For this review, use the dimensioned drawing (mm, ordinates from the lowest corner) and the shaded views. A direction names the side the tool comes from. Coordinates: 2 decimals unless noted, no trailing zeros. Loops run counter-clockwise (first coordinate to the right, second up) from the corner with the lowest first, then second, coordinate; pieces in that order, holes last. Notation, with made-up numbers: M 29.25,59.25 L 83.25,59.25 A24 cw 83.25,87.25 Z; hole C 45,83 d3. An arc over 180 degrees is marked long. Write item = value, one per line. Start each with the question number.
Q1. We need section A-A on y = 10.25. Give the boundary of the cut face in (x, z) (3 decimals).
Q2. For the marked faces 1 and 2, list the 3-axis set-ups (+Z, -Z, +X, -X, +Y, -Y) from which the entire face can be reached by the end or side of a thin tool; tool diameter is ignored.
Q3. Clearance check with flat-ended pins moving along their axes: pin 1 Ø5 at (y, z) = (5, 7.5) entering from +X; pin 2 Ø5 at (x, z) = (9.225, 9.225) entering from +Y; pin 3 Ø9 at (x, z) = (9, 13) entering from -Y; pin 4 Ø5 at (x, y) = (9.5, 8) entering from +Z. State where each tip first meets the part, or that it passes through.
Q4. Wall thickness on probe 1 along X at (y, z) = (12.75, 9.25); probe 2 along Y at (x, z) = (10, 4); probe 3 along Z at (x, y) = (9.5, 8): over which ranges is each line inside the solid? List them lowest first.
Q5. Mouldability with a two-part tool opening along X and no side actions: class the marked faces 3, 4 and 5 as released by +X, released by -X, zero draft, split by the parting line, or undercut.
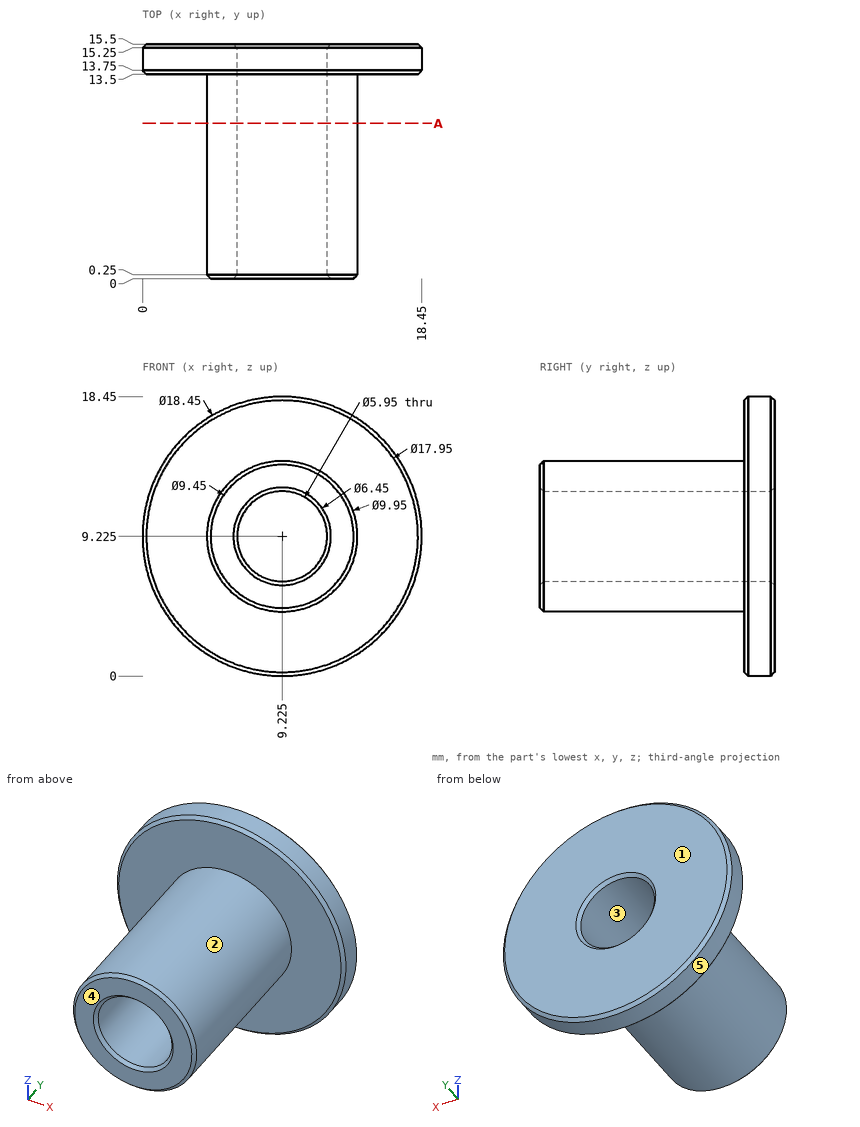
Returned:
q1.outline = C 9.225,9.225 d9.95; hole C 9.225,9.225 d5.95
q2.face_1 = +Z, -Z, +X, -X, +Y
q2.face_2 = -Y
q3.pin_1 = 14.2
q3.pin_2 = through
q3.pin_3 = 0
q3.pin_4 = 14.2
q4.probe_1 = 4.25 to 6.25, 12.2 to 14.2
q4.probe_2 = 13.5 to 15.5
q4.probe_3 = 4.26 to 6.26, 12.19 to 14.19
q5.face_3 = undercut
q5.face_4 = zero draft
q5.face_5 = split by the parting line
